```python
from build123d import *

# Parameters (mm, degrees)
F2_R     = 4.0538475773
F3_DEPTH = 8
F4_R     = 0.99999


# Not quite as in the source:
# - a fillet or chamfer is up to 0.001 mm smaller than in the source, because OpenCascade refuses the exact size


with BuildPart() as f1:
    # F0 (on Front) → F1 (revolve)
    with BuildSketch(Plane.XZ):
        Polygon((0, 4.0538475773), (0, 2.5), (5, 2.5), (5, 3.25), (8, 4.0538475773), align=None)
    revolve(axis=Axis((3.9731631987, 0, 0), (1, 0, 0)))

    # F2 (on Right) → F3 (join)
    with BuildSketch(Plane.YZ):
        with BuildLine():
            ThreePointArc((-2.2217503258, 5.8417741731), (-2.625, 4.5466333699), (-3.9482496742, 4.8449793096))
            ThreePointArc((-3.9482496742, 4.8449793096), (-4.4194173824, 4.4194173824), (-4.8449793096, 3.9482496742))
            ThreePointArc((-4.8449793096, 3.9482496742), (-4.5466333699, 2.625), (-5.8417741731, 2.2217503258))
            ThreePointArc((-5.8417741731, 2.2217503258), (-6.0370364143, 1.6176190319), (-6.17, 0.9967948636))
            ThreePointArc((-6.17, 0.9967948636), (-5.25, 0), (-6.17, -0.9967948636))
            ThreePointArc((-6.17, -0.9967948636), (-6.0370364143, -1.6176190319), (-5.8417741731, -2.2217503258))
            ThreePointArc((-5.8417741731, -2.2217503258), (-4.5466333699, -2.625), (-4.8449793096, -3.9482496742))
            ThreePointArc((-4.8449793096, -3.9482496742), (-4.4194173824, -4.4194173824), (-3.9482496742, -4.8449793096))
            ThreePointArc((-3.9482496742, -4.8449793096), (-2.625, -4.5466333699), (-2.2217503258, -5.8417741731))
            ThreePointArc((-2.2217503258, -5.8417741731), (-1.6176190319, -6.0370364143), (-0.9967948636, -6.17))
            ThreePointArc((-0.9967948636, -6.17), (0, -5.25), (0.9967948636, -6.17))
            ThreePointArc((0.9967948636, -6.17), (1.6176190319, -6.0370364143), (2.2217503258, -5.8417741731))
            ThreePointArc((2.2217503258, -5.8417741731), (2.625, -4.5466333699), (3.9482496742, -4.8449793096))
            ThreePointArc((3.9482496742, -4.8449793096), (4.4194173824, -4.4194173824), (4.8449793096, -3.9482496742))
            ThreePointArc((4.8449793096, -3.9482496742), (4.5466333699, -2.625), (5.8417741731, -2.2217503258))
            ThreePointArc((5.8417741731, -2.2217503258), (6.0370364143, -1.6176190319), (6.17, -0.9967948636))
            ThreePointArc((6.17, -0.9967948636), (5.25, 0), (6.17, 0.9967948636))
            ThreePointArc((6.17, 0.9967948636), (6.0370364143, 1.6176190319), (5.8417741731, 2.2217503258))
            ThreePointArc((5.8417741731, 2.2217503258), (4.5466333699, 2.625), (4.8449793096, 3.9482496742))
            ThreePointArc((4.8449793096, 3.9482496742), (4.4194173824, 4.4194173824), (3.9482496742, 4.8449793096))
            ThreePointArc((3.9482496742, 4.8449793096), (2.625, 4.5466333699), (2.2217503258, 5.8417741731))
            ThreePointArc((2.2217503258, 5.8417741731), (1.6176190319, 6.0370364143), (0.9967948636, 6.17))
            ThreePointArc((0.9967948636, 6.17), (0, 5.25), (-0.9967948636, 6.17))
            ThreePointArc((-0.9967948636, 6.17), (-1.6176190319, 6.0370364143), (-2.2217503258, 5.8417741731))
        make_face()
        Circle(F2_R, mode=Mode.SUBTRACT)
    extrude(amount=F3_DEPTH)

    # F4 (radius 1 in the source; OpenCascade refuses exactly that, so slightly less here)
    f4_edges = [f1.edges().sort_by_distance(p)[0] for p in [
        (8, -4.419417, 4.419417),
        (8, -1.617619, 6.037036),
        (8, 1.617619, 6.037036),
        (8, 4.419417, 4.419417),
        (8, 6.037036, 1.617619),
        (8, 6.037036, -1.617619),
        (8, 4.419417, -4.419417),
        (8, 1.617619, -6.037036),
        (8, -1.617619, -6.037036),
        (8, -4.419417, -4.419417),
        (8, -6.037036, -1.617619),
        (8, -6.037036, 1.617619),
    ]]
    fillet(f4_edges, radius=F4_R)


solid = f1.part
```
Part model, mm, in its own coordinate system. Round coordinates to 2 decimals unless told otherwise and drop trailing zeros. Loops run counter-clockwise (first coordinate to the right, second up) from the corner with the lowest first, then second, coordinate; pieces in that order, holes last.
1. Slice it at B-B (x = 6). Give the cut face in (y, z) (3 decimals), and give its area (3 significant figures).
Solutions:
outline: (-6.17, -0.997) arc R6.25 ccw to (-5.842, -2.222) arc R1 cw to (-4.845, -3.948) arc R6.25 ccw to (-3.948, -4.845) arc R1 cw to (-2.222, -5.842) arc R6.25 ccw to (-0.997, -6.17) arc R1 cw to (0.997, -6.17) arc R6.25 ccw to (2.222, -5.842) arc R1 cw to (3.948, -4.845) arc R6.25 ccw to (4.845, -3.948) arc R1 cw to (5.842, -2.222) arc R6.25 ccw to (6.17, -0.997) arc R1 cw to (6.17, 0.997) arc R6.25 ccw to (5.842, 2.222) arc R1 cw to (4.845, 3.948) arc R6.25 ccw to (3.948, 4.845) arc R1 cw to (2.222, 5.842) arc R6.25 ccw to (0.997, 6.17) arc R1 cw to (-0.997, 6.17) arc R6.25 ccw to (-2.222, 5.842) arc R1 cw to (-3.948, 4.845) arc R6.25 ccw to (-4.845, 3.948) arc R1 cw to (-5.842, 2.222) arc R6.25 ccw to (-6.17, 0.997) arc R1 cw to start; hole circle Ø7.036 at (0, 0)
area: 65.6 mm2
2. Two-plate mould, pull along Y, no slides. Class faces 1 (the face through (3.451, 1.626, 6.035)), 2 (the face through (3.944, 2.607, -4.557)), 3 (the face through (3.45, -4.43, -4.41)), 4 (the face through (8, 3, -3)): pulls with the +Y half, pulls with the -Y half, needs draft (parallel to the pull), parting line crosses it, or undercut.
Solutions:
face 1: pulls with the +Y half
face 2: undercut
face 3: pulls with the -Y half
face 4: needs draft
3. Flat gauge pins, fed straight in: pin 1 (1 mm diameter, centred on x = 7, z = 3.5, fed in from -Y) (3 decimals); pin 2 (2 mm diameter, centred on x = 1, z = -2.5, fed in from +Y). Where does each tip first touch, or does it go through?
Solutions:
pin 1: stops at y = -4.845
pin 2: stops at y = 6.07
4. Drill centre lines: line 1 along Z through (x, y) = (1.4, 0); line 2 along Y through (x, z) = (5.5, 2.5). Where is each one in solid material? Low to high.
Solutions:
line 1: z = -5.25 to -2.5, 2.5 to 5.25
line 2: y = -4.63 to -2.28, 2.28 to 4.63
5. Slice it at A-A (x = 2.25). Give the cut face in (y, z) (3 decimals), and give its area (3 significant figures).
Solutions:
outline: (-6.17, -0.997) arc R6.25 ccw to (-5.842, -2.222) arc R1 cw to (-4.845, -3.948) arc R6.25 ccw to (-3.948, -4.845) arc R1 cw to (-2.222, -5.842) arc R6.25 ccw to (-0.997, -6.17) arc R1 cw to (0.997, -6.17) arc R6.25 ccw to (2.222, -5.842) arc R1 cw to (3.948, -4.845) arc R6.25 ccw to (4.845, -3.948) arc R1 cw to (5.842, -2.222) arc R6.25 ccw to (6.17, -0.997) arc R1 cw to (6.17, 0.997) arc R6.25 ccw to (5.842, 2.222) arc R1 cw to (4.845, 3.948) arc R6.25 ccw to (3.948, 4.845) arc R1 cw to (2.222, 5.842) arc R6.25 ccw to (0.997, 6.17) arc R1 cw to (-0.997, 6.17) arc R6.25 ccw to (-2.222, 5.842) arc R1 cw to (-3.948, 4.845) arc R6.25 ccw to (-4.845, 3.948) arc R1 cw to (-5.842, 2.222) arc R6.25 ccw to (-6.17, 0.997) arc R1 cw to start; hole circle Ø5 at (0, 0)
area: 84.9 mm2
